Can you work these out from the model? Positions are in its coordinate system, mm. A direction names the side the tool comes from. Coordinates: 2 decimals unless noted, no trailing zeros. Write each loop counter-clockwise with the first axis right and the second up, starting at its lowest first coordinate (ties: lowest second). Pieces come first, ordered by that corner, then holes. Notation, with made-up numbers: (39, 10) - (96, 10) arc R28 cw to (96, 39) - close; hole circle Ø7 at (-27.75, 9). An arc over 180 degrees is marked (long way). Use one line per item in the form item = value. Start each with the question number.
(1) If we section it at D-D on y = -25.4: Please give me the cut outline in (x, z) (3 decimals).
(2) Thinking about a two-plate mould opening in Z: for faces 4 (the face through (0, -38.1, 14)), 5 (the face through (0.2, -11, -11.2)), 6 (the face through (0, -9.525, 0)), 7 (the face through (0, -22, 15.875)), which applies, pulls with the +Z half, pulls with the -Z half, needs draft (parallel to the pull), parting line crosses it, or undercut?
(3) On a 3-axis mill with a long thin cutter (end or side, diameter ignored), from which of +Z, -Z, +X, -X, +Y, -Y can I reach the whole of each face in a straight line? I mean faces 1 (the face through (12.7, -9, -4)), 2 (the face through (-12.7, -9, -4)), 3 (the face through (0, -29, 12.7)). Say none if no direction works.
(4) If we section it at C-C on x = 0: Give the number of separate pieces and of enclosed holes in the cut face, then the cut area to 3 significant figures.
(5) If we section it at A-A on y = -20.5: Please give me the cut outline in (x, z) (3 decimals), then the cut area to 3 significant figures.
(6) If I drill on probe 1 along Z at (x, y) = (0, -4.5); probe 2 along X at (y, z) = (-2, 38); probe 3 along Z at (x, y) = (1, -22) (3 decimals), over which ranges is the centre line in solid material (lowest first)? Write a range as from..to.
(7) If we section it at B-B on z = 38.1: Please give me the cut outline in (x, y).
(8) For pin 1 Ø3 at (x, z) = (13, 20) entering from -Y; pin 2 Ø8.5 at (x, y) = (0, -25.4) entering from -Z (3 decimals); pin 3 Ø2 at (x, y) = (6.5, -32) entering from +Z (3 decimals); pin 4 Ø5 at (x, y) = (0, -25.4) entering from -Z, each with a flat end and sliding along its axis, tell me the tip position at first contact or that it passes through.
```python
from build123d import *

# Parameters (mm, degrees)
F0_W     = 50.8
F0_H     = 101.6
F0_R     = 3.302
F1_DEPTH = 6.35
F2_W     = 25.4
F2_H     = 3.175
F3_DEPTH = 31.75
F2_H_2   = 25.4
F4_DEPTH = 3.175
F5_R     = 5.08
F6_R     = 5.08
F7_R     = 3.175
F8_DEPTH = 66.676


with BuildPart() as f1:
    # F0 (on Front) → F1 (new body)
    with BuildSketch(Plane.XZ):
        Rectangle(F0_W, F0_H)
        with Locations((0, -38.1)):
            Circle(F0_R, mode=Mode.SUBTRACT)
        with Locations((0, 38.1)):
            Circle(F0_R, mode=Mode.SUBTRACT)
    extrude(amount=F1_DEPTH)

    # F2 (on face) → F3 (join)
    with BuildSketch(Plane.XZ.offset(6.35)):
        with Locations((0, -14.2875)):
            Rectangle(F2_W, F2_H)
        with Locations((0, 14.2875)):
            Rectangle(F2_W, F2_H)
    extrude(amount=F3_DEPTH)

    # F2 (on face) → F4 (join)
    with BuildSketch(Plane.XZ.offset(6.35)):
        with Locations((0, 14.2875)):
            Rectangle(F2_W, F2_H)
        Rectangle(F2_W, F2_H_2)
        with Locations((0, -14.2875)):
            Rectangle(F2_W, F2_H)
    extrude(amount=F4_DEPTH)

    # F5
    f5_edges = [f1.edges().sort_by_distance(p)[0] for p in [
        (0, -9.525, -12.7),
        (0, -9.525, 12.7),
    ]]
    fillet(f5_edges, radius=F5_R)

    # F6
    f6_edges = [f1.edges().sort_by_distance(p)[0] for p in [
        (12.7, -38.1, 14.2875),
        (-12.7, -38.1, 14.2875),
        (12.7, -38.1, -14.2875),
        (-12.7, -38.1, -14.2875),
    ]]
    fillet(f6_edges, radius=F6_R)

    # F7 (on face) → F8 (cut, through all)
    with BuildSketch(Plane.XY.offset(15.875)):
        with Locations((0, -25.4)):
            Circle(F7_R)
    extrude(amount=-F8_DEPTH, mode=Mode.SUBTRACT)


solid = f1.part
```
Reported:
q1.outline = (-12.7, -15.875) - (-3.175, -15.875) - (-3.175, -12.7) - (-12.7, -12.7) - close; (-12.7, 12.7) - (-3.175, 12.7) - (-3.175, 15.875) - (-12.7, 15.875) - close; (3.175, -15.875) - (12.7, -15.875) - (12.7, -12.7) - (3.175, -12.7) - close; (3.175, 12.7) - (12.7, 12.7) - (12.7, 15.875) - (3.175, 15.875) - close
q2.face_4 = needs draft
q2.face_5 = undercut
q2.face_6 = undercut
q2.face_7 = pulls with the +Z half
q3.face_1 = +Z, -Z, +X, -Y
q3.face_2 = +Z, -Z, -X, -Y
q3.face_3 = +X, -X, -Y
q4.separate_pieces = 5
q4.enclosed_holes = 0
q4.area = 814 mm2
q5.outline = (-12.7, -15.875) - (12.7, -15.875) - (12.7, -12.7) - (-12.7, -12.7) - close; (-12.7, 12.7) - (12.7, 12.7) - (12.7, 15.875) - (-12.7, 15.875) - close
q5.area = 161 mm2
q6.probe_1 = -50.8..-41.4, -34.8..34.8, 41.4..50.8
q6.probe_2 = -25.4..-3.3, 3.3..25.4
q6.probe_3 = -15.875..-12.7, 12.7..15.875
q7.outline = (-25.4, -6.35) - (-3.3, -6.35) - (-3.3, 0) - (-25.4, 0) - close; (3.3, -6.35) - (25.4, -6.35) - (25.4, 0) - (3.3, 0) - close
q8.pin_1 = -6.35
q8.pin_2 = -15.875
q8.pin_3 = 15.875
q8.pin_4 = through
